Design review of the part shown in the three views and the two pictorial views. Dimensions are in mm from the part's minimum x, y and z. A direction names the side the tool comes from. Give positions to 0.01 mm unless a question says otherwise; leave off trailing zeros. Order: outer loops, then holes, each group sorted by start corner. A loop starts at its lowest first (then second) coordinate and runs counter-clockwise, first axis right, second up.
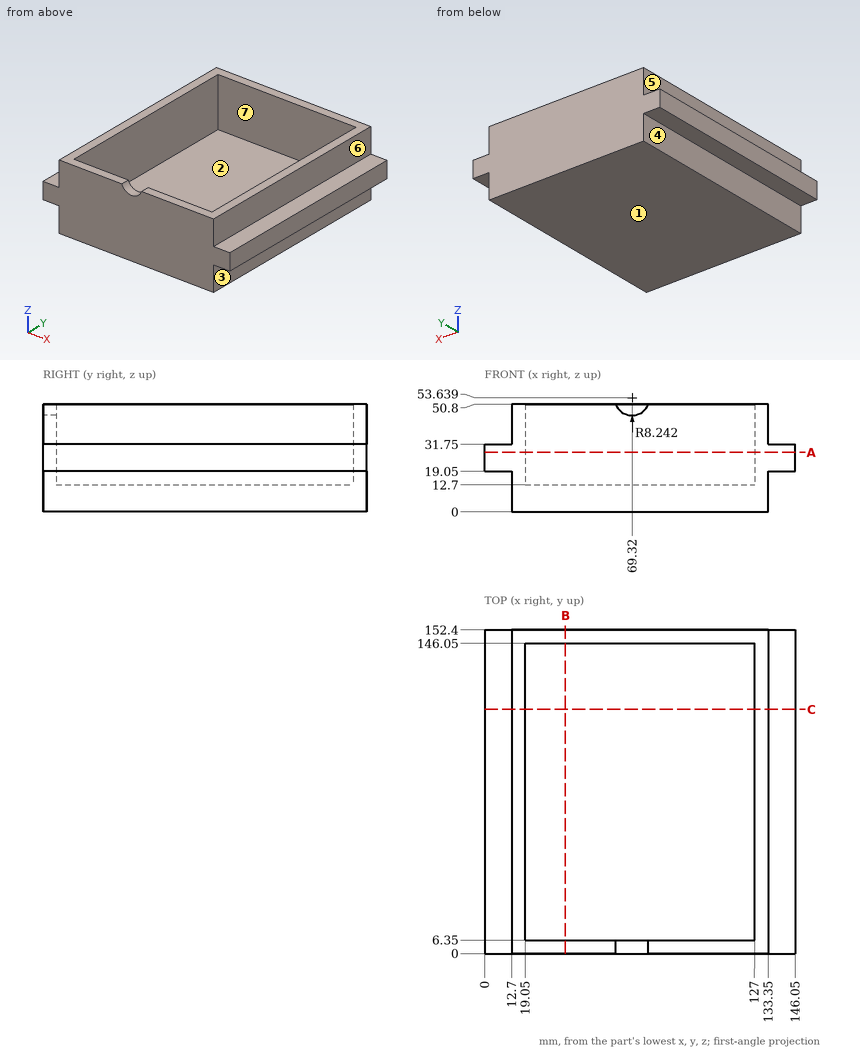
Item 1: For line 1 (X direction, y = 28, z = 17); line 2 (X direction, y = 106, z = 22); line 3 (Y direction, x = 103, z = 28), list the stretches that pass through material, from the lowest coordinate up.
Values found:
line 1: x = 12.7 to 19.05, 127 to 133.35
line 2: x = 0 to 19.05, 127 to 146.05
line 3: y = 0 to 6.35, 146.05 to 152.4
Item 2: Take a section at B-B (x = 38). Give the boundary of the cut face in (y, z).
Values found:
outline: (0, 0) - (152.4, 0) - (152.4, 50.8) - (146.05, 50.8) - (146.05, 12.7) - (6.35, 12.7) - (6.35, 50.8) - (0, 50.8) - close
Item 3: For the marked faces 4, 5, 6 and 7, list the 3-axis set-ups (+Z, -Z, +X, -X, +Y, -Y) from which the entire face can be reached by the end or side of a thin tool; tool diameter is ignored.
Values found:
face 4: -Z, -X, +Y, -Y
face 5: +Z, -X, +Y, -Y
face 6: +Z, +X, +Y, -Y
face 7: +Z
Item 4: Take a section at A-A (z = 28). Give the boundary of the cut face in (x, y), and give its area (3 significant figures).
Values found:
outline: (0, 0) - (146.05, 0) - (146.05, 152.4) - (0, 152.4) - close; hole (19.05, 6.35) - (127, 6.35) - (127, 146.05) - (19.05, 146.05) - close
area: 7,180 mm2
Item 5: Draft analysis for pull direction X (two halves, no side actions). For the marked faces 1, 2 and 3, state which applies: released by +X, released by -X, zero draft, split by the parting line, or undercut.
Values found:
face 1: zero draft
face 2: undercut
face 3: released by +X
Item 6: Clearance check with flat-ended pins moving along their axes: pin 1 Ø4 at (y, z) = (90, 5) entering from +X; pin 2 Ø9.5 at (y, z) = (70, 39.5) entering from -X; pin 3 Ø6 at (x, y) = (83.5, 48.5) entering from +Z. State where each tip first meets the part, or that it passes through.
Values found:
pin 1: stops at x = 133.35
pin 2: stops at x = 12.7
pin 3: stops at z = 12.7
Item 7: Take a section at C-C (y = 115). Give the boundary of the cut face in (x, z), and give its area (3 significant figures).
Values found:
outline: (0, 19.05) - (12.7, 19.05) - (12.7, 0) - (133.35, 0) - (133.35, 19.05) - (146.05, 19.05) - (146.05, 31.75) - (133.35, 31.75) - (133.35, 50.8) - (127, 50.8) - (127, 12.7) - (19.05, 12.7) - (19.05, 50.8) - (12.7, 50.8) - (12.7, 31.75) - (0, 31.75) - close
area: 2,340 mm2
